Input: part model. Units: mm. Frame: model coordinates. Face numbers are marked on the shaded views. Round coordinates to 2 decimals unless told otherwise and drop trailing zeros. Write each loop counter-clockwise with the first axis right and the second up, starting at its lowest first coordinate (ties: lowest second). Pieces come first, ordered by that corner, then holes. Notation, with made-up numbers: (-31.75, 4.5) - (9.25, 4.5) arc R13 cw to (9.25, 28.5) - close; hole circle Ø8 at (-1, -2.75). An arc over 180 degrees is marked (long way). Use one line per item in the form item = value.
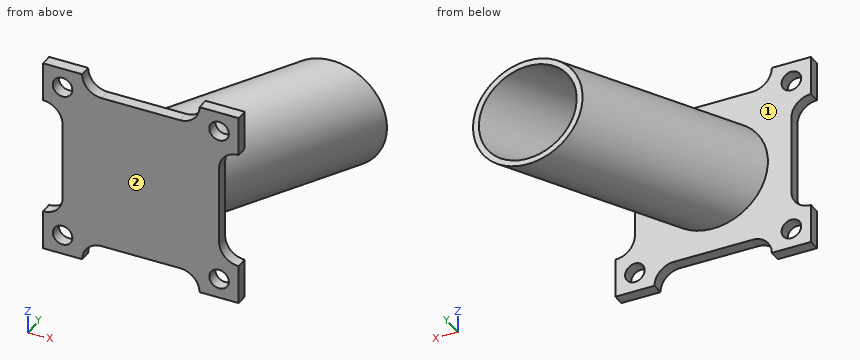
```python
from build123d import *

# Parameters (mm, degrees)
SKETCH1_W           = 50
SKETCH1_H           = 50
BOSS_EXTRUDE1_DEPTH = 3
SKETCH3_R           = 14
SKETCH3_R_2         = 12.5
CUT_EXTRUDE1_REACH  = 65.411
SKETCH4_R           = 2.5
CUT_EXTRUDE2_REACH  = 65.411
CIRPATTERN1_COUNT   = 4


with BuildPart() as part:
    # Sketch1 → Boss-Extrude1 (new body)
    with BuildSketch(Plane(origin=(0, 0, 0), x_dir=(1, 0, 0), z_dir=(0, 1, 0))):
        Rectangle(SKETCH1_W, SKETCH1_H)
    extrude(amount=BOSS_EXTRUDE1_DEPTH)

    # Sweep1: sweep along a path in Sketch2
    with BuildLine(Plane.XY) as sweep1_path:
        Line((0, 3), (25, 46.301270189))
    # Sketch3 → Sweep1 (sweep)
    with BuildSketch(Plane(origin=(0, 3, 0), x_dir=(1, 0, 0), z_dir=(0, 1, 0))):
        Circle(SKETCH3_R)
        Circle(SKETCH3_R_2, mode=Mode.SUBTRACT)
    sweep(path=sweep1_path.line)

    # Sketch4 → Cut-Extrude1 (cut, up to next)
    with BuildSketch(Plane(origin=(0, 3, 0), x_dir=(1, 0, 0), z_dir=(0, 1, 0)), mode=Mode.PRIVATE) as cut_extrude1_sk1:
        with Locations(Location((-20, 20, 0), (0, 0, 270))):
            Circle(SKETCH4_R)
    cut_extrude1_tool1 = extrude(cut_extrude1_sk1.sketch, amount=-CUT_EXTRUDE1_REACH, mode=Mode.PRIVATE) & part.part
    # Sketch4 → Cut-Extrude1 (cut, up to next)
    with BuildSketch(Plane(origin=(0, 3, 0), x_dir=(1, 0, 0), z_dir=(0, 1, 0)), mode=Mode.PRIVATE) as cut_extrude1_sk2:
        with Locations(Location((20, 20, 0), (0, 0, 270))):
            Circle(SKETCH4_R)
    cut_extrude1_tool2 = extrude(cut_extrude1_sk2.sketch, amount=-CUT_EXTRUDE1_REACH, mode=Mode.PRIVATE) & part.part
    # Sketch4 → Cut-Extrude1 (cut, up to next)
    with BuildSketch(Plane(origin=(0, 3, 0), x_dir=(1, 0, 0), z_dir=(0, 1, 0)), mode=Mode.PRIVATE) as cut_extrude1_sk3:
        with Locations(Location((20, -20, 0), (0, 0, 270))):
            Circle(SKETCH4_R)
    cut_extrude1_tool3 = extrude(cut_extrude1_sk3.sketch, amount=-CUT_EXTRUDE1_REACH, mode=Mode.PRIVATE) & part.part
    # Sketch4 → Cut-Extrude1 (cut, up to next)
    with BuildSketch(Plane(origin=(0, 3, 0), x_dir=(1, 0, 0), z_dir=(0, 1, 0)), mode=Mode.PRIVATE) as cut_extrude1_sk4:
        with Locations(Location((-20, -20, 0), (0, 0, 270))):
            Circle(SKETCH4_R)
    cut_extrude1_tool4 = extrude(cut_extrude1_sk4.sketch, amount=-CUT_EXTRUDE1_REACH, mode=Mode.PRIVATE) & part.part
    add(cut_extrude1_tool1.solids().sort_by_distance((-20, 3, -20))[0], mode=Mode.SUBTRACT)
    add(cut_extrude1_tool2.solids().sort_by_distance((20, 3, -20))[0], mode=Mode.SUBTRACT)
    add(cut_extrude1_tool3.solids().sort_by_distance((20, 3, 20))[0], mode=Mode.SUBTRACT)
    add(cut_extrude1_tool4.solids().sort_by_distance((-20, 3, 20))[0], mode=Mode.SUBTRACT)

    # Sketch5 → Cut-Extrude2 (cut, up to next)
    with BuildSketch(Plane(origin=(0, 3, 0), x_dir=(1, 0, 0), z_dir=(0, 1, 0)), mode=Mode.PRIVATE) as cut_extrude2_sk1:
        with BuildLine():
            Line((-10, 30), (10, 30))
            ThreePointArc((10, 30), (15, 25), (10, 20))
            Line((10, 20), (-10, 20))
            ThreePointArc((-10, 20), (-15, 25), (-10, 30))
        make_face()
    cut_extrude2_tool1 = extrude(cut_extrude2_sk1.sketch, amount=-CUT_EXTRUDE2_REACH, mode=Mode.PRIVATE) & part.part
    cut_extrude2 = cut_extrude2_tool1.solids().sort_by_distance((0, 3, -25))[0]
    add(cut_extrude2, mode=Mode.SUBTRACT)

    # CirPattern1: Cut-Extrude2 ×4 about axis
    cirpattern1_axis = Axis((0, 0, 0), (0, 1, 0))
    for i in range(1, CIRPATTERN1_COUNT):
        add(cut_extrude2.rotate(cirpattern1_axis, i * 360 / CIRPATTERN1_COUNT), mode=Mode.SUBTRACT)


solid = part.part
```
(1) First-contact query: pin 1 Ø1.5 at (y, z) = (2, 21) entering from +X; pin 2 Ø4 at (x, y) = (14, 12) entering from -Z; pin 3 Ø20 at (x, z) = (-3.5, -4) entering from +Y. Flat tips, straight axial feed; report the tip coordinate or a pass-through.
Derived:
pin_1 = 25
pin_2 = -12.4
pin_3 = 37.93
(2) Cut plane A-A on z = 16. Output: boundary loops of the cut face in (x, y).
Derived:
outline = (-25, 0) - (25, 0) - (25, 3) - (-25, 3) - close
(3) Draft query along Y for the marked faces 1 and 2. Return one class per face: released by +Y, released by -Y, zero draft, split by the parting line, or undercut.
Derived:
face_1 = undercut
face_2 = released by -Y
(4) Material intervals for L1, parallel to Z at x = 16.5, y = 32.5; L2, parallel to Y at x = -14, z = 5; L3, parallel to X at y = 19, z = 9, sorted ascending.
Derived:
L1 = -13.99 to -12.49, 12.49 to 13.99
L2 = 0 to 3
L3 = -1.49 to 0.56, 17.91 to 19.96
